Build history of the part. All positions in model axes, mm. A direction names the side the tool comes from. Coordinates: 2 decimals unless noted, no trailing zeros. Write each loop counter-clockwise with the first axis right and the second up, starting at its lowest first coordinate (ties: lowest second). Pieces come first, ordered by that corner, then holes.
```python
from build123d import *

# Parameters (mm, degrees)
SKETCH1_R           = 1.5
BOSS_EXTRUDE1_DEPTH = 10
REVOLVE1_ANGLE      = 180
CUT_EXTRUDE1_DEPTH  = 2


with BuildPart() as part:
    # Sketch1 → Boss-Extrude1 (new body)
    with BuildSketch(Plane.XY):
        Circle(SKETCH1_R)
    extrude(amount=BOSS_EXTRUDE1_DEPTH)

    # Sketch2 → Revolve1 (revolve)
    with BuildSketch(Plane.XY.offset(10)):
        with BuildLine():
            Line((0, 2.5), (0, -2.5))
            ThreePointArc((0, -2.5), (2.5, 0), (0, 2.5))
        make_face()
    revolve(axis=Axis((0, 2.5, 10), (0, -1, 0)), revolution_arc=REVOLVE1_ANGLE)

    # Sketch3 → Cut-Extrude1 (cut)
    with BuildSketch(Plane.XY.offset(13)):
        Polygon((0.5, 0.5), (3, 0.5), (3, -0.5), (0.5, -0.5), (0.5, -3.070620821), (-0.5, -3.070620821), (-0.5, -0.5), (-3, -0.5), (-3, 0.5), (-0.5, 0.5), (-0.5, 2.929379179), (0.5, 2.929379179), align=None)
    extrude(amount=-CUT_EXTRUDE1_DEPTH, mode=Mode.SUBTRACT)


solid = part.part
```
1. Flat gauge pins, fed straight in: pin 1 (0.7 mm diameter, centred on x = 1.5, z = 11.5, fed in from +Y); pin 2 (1.5 mm diameter, centred on x = -1, z = 12, fed in from +Y); pin 3 (0.7 mm diameter, centred on y = 1.5, z = 11.5, fed in from +X). Where does each tip first touch, or does it go through?
Computed values:
pin 1: stops at y = 1.76
pin 2: stops at y = 2.01
pin 3: stops at x = 1.76
2. Saw through at C-C on z = 1.25. List the corners of the cut face in (x, y), plus the area to 3 significant figures.
Computed values:
outline: circle Ø3 at (0, 0)
area: 7.07 mm2
3. Saw through at D-D on x = -2.05. List the corners of the cut face in (y, z).
Computed values:
outline: (-1.43, 10) - (1.43, 10) arc R1.43 ccw to (0.5, 11.34) - (0.5, 11) - (-0.5, 11) - (-0.5, 11.34) arc R1.43 ccw to start
4. 3-axis set-ups, long thin cutter, end or side, ignore diameter. For faces 1 (the face through (2, 0, 10)), 2 (the face through (-1, -0.5, 12)), 3 (the face through (0.5, -1, 12)): which of +Z, -Z, +X, -X, +Y, -Y reach the whole face in a straight line?
Computed values:
face 1: -Z
face 2: +Z, +X, -X
face 3: +Z, +Y, -Y
5. Probe line 1 along Z through (x, y) = (0.1, -2.25); line 2 along X through (y, z) = (0.85, 11.25); line 3 along Z through (x, y) = (-0.4, 0.6). List the from-to ranges inside material, lowest first.
Computed values:
line 1: z = 10 to 11
line 2: x = -1.99 to -0.5, 0.5 to 1.99
line 3: z = 0 to 11
6. Saw through at A-A on y = 0. List the corners of the cut face in (x, z).
Computed values:
outline: (-2.5, 10) - (-1.5, 10) - (-1.5, 0) - (1.5, 0) - (1.5, 10) - (2.5, 10) arc R2.5 ccw to (2.29, 11) - (-2.29, 11) arc R2.5 ccw to start
7. Mould opens along X. For faces 4 (the face through (1, 0.5, 12)), 5 (the face through (0.5, 1, 12)), 6 (the face through (-0.5, 1, 12)), 7 (the face through (-1.5, 0.07, 4.93)) say: +X half, -X half, draft (parallel to the pull), parting line (faces both ways), or undercut.
Computed values:
face 4: draft
face 5: undercut
face 6: undercut
face 7: parting line
